Source: CAD feature listing. Evaluate the final solid. Frame: model axes, mm. Face numbers are marked on the shaded views. A direction names the side the tool comes from. Round coordinates to 2 decimals unless told otherwise and drop trailing zeros. Loops run counter-clockwise (first coordinate to the right, second up) from the corner with the lowest first, then second, coordinate; pieces in that order, holes last.
Item 1: Section query A-A on y = 0. Return loops of the section in (x, z).
Item 2: Ray query, L1, parallel to X at y = 0, z = 6.5; L2, parallel to X at y = 0, z = 0.6; L3, parallel to Y at x = 0, z = 1. Return the intervals inside material, ascending.
Item 3: Section query C-C on z = 5. Return loops of the section in (x, y).
Item 4: Section query B-B on x = 15. Return loops of the section in (y, z), then the cut area to 4 significant figures.
Item 5: Access query for the marked faces 1, 2 and 3. Directions: +Z, -Z, +X, -X, +Y, -Y. A direction counts if a zero-diameter tool reaches every point of the face in a straight line with its end or side. Return the directions, or none.
Item 6: First-contact query: P1, Ø9.5, axis at x = 15, y = 0, coming from the -Z side; P2, Ø5, axis at x = 12, z = 6.5, coming from the -Y side; P3, Ø1, axis at x = 5, z = 8, coming from the -Y side. Flat tips, straight axial feed; report the tip coordinate or a pass-through.
Item 7: Pull-direction query (Y, two-part tool) for the marked faces 4, 5 and 6; classes: released by +Y, released by -Y, zero draft, split by the parting line, or undercut.
```python
from build123d import *

# Parameters (mm, degrees)
SKETCH_R        = 2.1
SKETCH_R_2      = 1.5
PAD_DEPTH       = 10
POCKET_DEPTH    = 3
SKETCH002_R     = 2.1
SKETCH002_R_2   = 1.5
PAD001_DEPTH    = 2
SKETCH003_R     = 3.6
SKETCH003_R_2   = 2.1
POCKET001_DEPTH = 2.5
FILLET_R        = 1
FILLET001_R     = 5
SKETCH004_R     = 1.5
PAD002_DEPTH    = 0.1


with BuildPart() as part:
    # Sketch → Pad (new body)
    with BuildSketch(Plane.XY):
        with BuildLine():
            Line((-22.5, 10), (22.5, 10))
            Line((22.5, 10), (22.5, -10))
            Line((22.5, -10), (6, -10))
            Line((6, -15), (6, -10))
            ThreePointArc((-6, -15), (0, -21), (6, -15))
            Line((-6, -15), (-6, -10))
            Line((-22.5, -10), (-6, -10))
            Line((-22.5, -10), (-22.5, 10))
        make_face()
        with Locations((-15, 0)):
            Circle(SKETCH_R, mode=Mode.SUBTRACT)
        with Locations((15, 0)):
            Circle(SKETCH_R, mode=Mode.SUBTRACT)
        with Locations((0, 5)):
            Circle(SKETCH_R_2, mode=Mode.SUBTRACT)
        with Locations((0, -15)):
            Circle(SKETCH_R_2, mode=Mode.SUBTRACT)
    extrude(amount=PAD_DEPTH)

    # Sketch001 → Pocket (cut)
    with BuildSketch(Plane.XY.offset(10)):
        Polygon((1.587713, 2.25), (3.175426, 5), (1.587713, 7.75), (-1.587713, 7.75), (-3.175426, 5), (-1.587713, 2.25), align=None)
        Polygon((1.587713, -17.75), (3.175426, -15), (1.587713, -12.25), (-1.587713, -12.25), (-3.175426, -15), (-1.587713, -17.75), align=None)
    extrude(amount=-POCKET_DEPTH, mode=Mode.SUBTRACT)

    # Sketch002 → Pad001 (new body)
    with BuildSketch(Plane(origin=(0, 0, 0), x_dir=(1, 0, 0), z_dir=(0, 0, -1))):
        with Locations((0, -5)):
            Circle(SKETCH002_R)
        with Locations((0, -5)):
            Circle(SKETCH002_R_2, mode=Mode.SUBTRACT)
        with Locations((0, 15)):
            Circle(SKETCH002_R)
        with Locations((0, 15)):
            Circle(SKETCH002_R_2, mode=Mode.SUBTRACT)
    extrude(amount=PAD001_DEPTH)

    # Sketch003 → Pocket001 (cut)
    with BuildSketch(Plane(origin=(0, 0, 0), x_dir=(1, 0, 0), z_dir=(0, 0, -1))):
        with Locations((15, 0)):
            Circle(SKETCH003_R)
        with Locations((15, 0)):
            Circle(SKETCH003_R_2, mode=Mode.SUBTRACT)
        with Locations((-15, 0)):
            Circle(SKETCH003_R)
        with Locations((-15, 0)):
            Circle(SKETCH003_R_2, mode=Mode.SUBTRACT)
    extrude(amount=-POCKET001_DEPTH, mode=Mode.SUBTRACT)

    # Fillet
    fillet_edges = [part.edges().sort_by_distance(p)[0] for p in [
        (-2.1, 5, 0),
        (-2.1, -15, 0),
    ]]
    fillet(fillet_edges, radius=FILLET_R)

    # Fillet001
    fillet001_edges = [part.edges().sort_by_distance(p)[0] for p in [
        (22.5, 10, 5),
        (22.5, -10, 5),
        (-22.5, 10, 5),
        (-22.5, -10, 5),
    ]]
    fillet(fillet001_edges, radius=FILLET001_R)

    # Sketch004 → Pad002 (new body)
    with BuildSketch(Plane.XY.offset(7)):
        with Locations((0, 5)):
            Circle(SKETCH004_R)
        with Locations((0, -15)):
            Circle(SKETCH004_R)
    extrude(amount=-PAD002_DEPTH)


solid = part.part
```
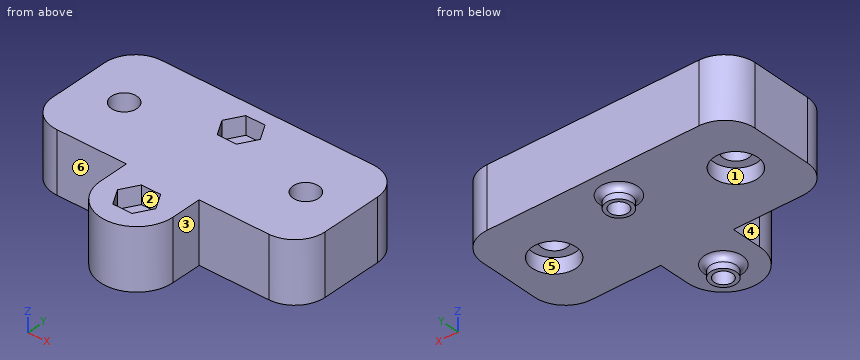
Data:
1. outline: (-22.5, 0) - (-18.6, 0) - (-18.6, 2.5) - (-17.1, 2.5) - (-17.1, 10) - (-22.5, 10) - close; (-12.9, 2.5) - (-11.4, 2.5) - (-11.4, 0) - (11.4, 0) - (11.4, 2.5) - (12.9, 2.5) - (12.9, 10) - (-12.9, 10) - close; (17.1, 2.5) - (18.6, 2.5) - (18.6, 0) - (22.5, 0) - (22.5, 10) - (17.1, 10) - close
2. L1: x = -22.5 to -17.1, -12.9 to 12.9, 17.1 to 22.5
2. L2: x = -22.5 to -18.6, -11.4 to 11.4, 18.6 to 22.5
2. L3: y = -21 to -16.5, -13.5 to 3.5, 6.5 to 10
3. outline: (-22.5, -5) arc R5 ccw to (-17.5, -10) - (-6, -10) - (-6, -15) arc R6 ccw to (6, -15) - (6, -10) - (17.5, -10) arc R5 ccw to (22.5, -5) - (22.5, 5) arc R5 ccw to (17.5, 10) - (-17.5, 10) arc R5 ccw to (-22.5, 5) - close; hole circle Ø4.2 at (-15, 0); hole circle Ø3 at (0, -15); hole circle Ø3 at (0, 5); hole circle Ø4.2 at (15, 0)
4. outline: (-10, 0) - (-3.6, 0) - (-3.6, 2.5) - (-2.1, 2.5) - (-2.1, 10) - (-10, 10) - close; (2.1, 2.5) - (3.6, 2.5) - (3.6, 0) - (10, 0) - (10, 10) - (2.1, 10) - close
4. area: 150.5 mm2
5. face 1: -Z
5. face 2: +Z
5. face 3: +Z, -Z, +X, -Y
6. P1: stops at z = 0
6. P2: stops at y = -10
6. P3: stops at y = -18.97
7. face 4: zero draft
7. face 5: undercut
7. face 6: released by -Y
